Can you work these out from the model? Positions are in its coordinate system, mm. A direction names the side the tool comes from. Give positions to 0.01 mm unless a question says otherwise; leave off trailing zeros. Loops run counter-clockwise (first coordinate to the right, second up) from the corner with the lowest first, then second, coordinate; pieces in that order, holes last. Notation, with made-up numbers: M 0.25,12.25 L 51.25,12.25 A9 ccw 51.25,25.25 Z; hole C -5.75,-2.75 d10. An arc over 180 degrees is marked long. Use CSV: the item, a comma, the result in double quotes.
from build123d import *

# Parameters (mm, degrees)
F1_DEPTH = 51.5
F2_W     = 10
F2_H     = 8.67
F3_DEPTH = 51.501
F5_DEPTH = 13
F6_W     = 13
F6_H     = 3
F7_DEPTH = 5


with BuildPart() as f1:
    # F0 (on Front) → F1 (new body)
    with BuildSketch(Plane.XZ):
        Polygon((-9.96814, 13.299286), (-29.225, -13.49947), (29.775, -13.49947), (10.51814, 13.299286), align=None)
    extrude(amount=F1_DEPTH)

    # F2 (on face) → F3 (cut, through all)
    with BuildSketch(Plane.XZ.offset(51.5)):
        with Locations((0.275, -9.16447)):
            Rectangle(F2_W, F2_H)
    extrude(amount=-F3_DEPTH, mode=Mode.SUBTRACT)

    # F4 (on face) → F5 (cut)
    with BuildSketch(Plane.XZ.offset(51.5)):
        Polygon((-6.187351, -8.99947), (-4.725, -8.99947), (-4.725, -4.82947), (5.275, -4.82947), (5.275, -8.99947), (6.812649, -8.99947), (6.812649, 13.299286), (-6.187351, 13.299286), align=None)
    extrude(amount=-F5_DEPTH, mode=Mode.SUBTRACT)

    # F6 (on face) → F7 (cut)
    with BuildSketch(Plane.XZ.offset(38.5)):
        with Locations((0.312649, 9.799286)):
            Rectangle(F6_W, F6_H)
    extrude(amount=-F7_DEPTH, mode=Mode.SUBTRACT)


solid = f1.part
Q1. I want a section at A-A, the plane y = -40. Please give me the cut outline in (x, z) (3 decimals), then the cut area to 3 significant figures.
Model answer:
outline,"M -29.225,-13.499 L -4.725,-13.499 L -4.725,-8.999 L -6.187,-8.999 L -6.187,13.299 L -9.968,13.299 Z; M 5.275,-13.499 L 29.775,-13.499 L 10.518,13.299 L 6.813,13.299 L 6.813,-8.999 L 5.275,-8.999 Z"
area,"730 mm2"
Q2. I'm going to push flat-ended pins straight in: P1, Ø10, axis at x = -20.5, y = -27.5, coming from the +Z side; P2, Ø1.5, axis at x = 0, y = -35, coming from the -Z side; P3, Ø2, axis at x = -2, z = 12.5, coming from the -Y side. Where does each tip first touch, or does it pass through?
Model answer:
P1,"z = 5.6"
P2,"z = -4.83"
P3,"y = -38.5"
Q3. If we mould it in two halves opening along Z, with no side actions, what happens to faces 6 (the flat face through (20.281, -25.39, -0.288)), 7 (the flat face through (0, -36, 11.299)), 8 (the flat face through (5.275, -26, -9))? For each: released by +Z, released by -Z, zero draft, split by the parting line, or undercut.
Model answer:
face 6,"released by +Z"
face 7,"undercut"
face 8,"zero draft"
Q4. I want a section at B-B, the plane z = -8.25. Please give me the cut outline in (x, y) (3 decimals), then the cut area to 3 significant figures.
Model answer:
outline,"M -25.453,-51.5 L -6.187,-51.5 L -6.187,-38.5 L -4.725,-38.5 L -4.725,0 L -25.453,0 Z; M 5.275,-38.5 L 6.813,-38.5 L 6.813,-51.5 L 26.003,-51.5 L 26.003,0 L 5.275,0 Z"
area,"2,100 mm2"
Q5. Please list where these lines run through material, in increasing order: L1, parallel to Y at x = -5, z = 5.5; L2, parallel to Z at x = -4, y = -7; L3, parallel to X at y = -29.5, z = -5.25 (3 decimals). Write a range as from..to.
Model answer:
L1,"-38.5..0"
L2,"-4.83..13.3"
L3,"-23.297..-4.725, 5.275..23.847"
Q6. For faces 1 (the flat face through (6, -45, -8.999)), 2 (the flat face through (-4.725, -26, -9)), 3 (the flat face through (0, -36, 8.299)), 4 (the flat face through (0, 0, -3)), 5 (the flat face through (-17, -25, -13.499)), which set-ups out of +Z, -Z, +X, -X, +Y, -Y let a thin tool reach every point of the face, with its end or its side?
Model answer:
face 1,"+Z, -Y"
face 2,"-Z, +Y, -Y"
face 3,"-Y"
face 4,"+Z, -Z, +X, -X, +Y"
face 5,"-Z, +X, -X, +Y, -Y"
Q7. I want a section at C-C, the plane x = 1. Please give me the cut outline in (y, z).
Model answer:
outline,"M -38.5,-4.83 L 0,-4.83 L 0,13.3 L -38.5,13.3 L -38.5,11.3 L -33.5,11.3 L -33.5,8.3 L -38.5,8.3 Z"
Q8. I want a section at D-D, the plane y = -23. Please give me the cut outline in (x, z) (3 decimals), then the cut area to 3 significant figures.
Model answer:
outline,"M -29.225,-13.499 L -4.725,-13.499 L -4.725,-4.829 L 5.275,-4.829 L 5.275,-13.499 L 29.775,-13.499 L 10.518,13.299 L -9.968,13.299 Z"
area,"978 mm2"
